from build123d import *

# Parameters (mm, degrees)
SKETCH1_R           = 101.6
SKETCH1_R_2         = 98.425
BOSS_EXTRUDE1_DEPTH = 152.4
CUT_EXTRUDE1_DEPTH  = 152.4
FILLET1_R           = 12.7


with BuildPart() as part:
    # Sketch1 → Boss-Extrude1 (new body)
    with BuildSketch(Plane(origin=(0, 0, 0), x_dir=(1, 0, 0), z_dir=(0, 1, 0))):
        Circle(SKETCH1_R)
        Circle(SKETCH1_R_2, mode=Mode.SUBTRACT)
    extrude(amount=BOSS_EXTRUDE1_DEPTH)

    # Sketch2 → Cut-Extrude1 (cut)
    with BuildSketch(Plane(origin=(0, 0, 0), x_dir=(1, 0, 0), z_dir=(0, 1, 0))):
        Polygon((570.652570484, -39.903914981), (101.352507506, -7.087257732), (0, 0), (-101.352507506, -7.087257732), (-570.652570484, -39.903914981), (-570.652570484, -980.796006784), (570.652570484, -980.796006784), align=None)
    extrude(amount=CUT_EXTRUDE1_DEPTH, mode=Mode.SUBTRACT)

    # Fillet1
    fillet1_edges = [part.edges().sort_by_distance(p)[0] for p in [
        (-99.768874577, 0, 6.97651933),
        (99.768874577, 152.4, 6.97651933),
        (-99.768874577, 152.4, 6.97651933),
        (99.768874577, 0, 6.97651933),
    ]]
    fillet(fillet1_edges, radius=FILLET1_R)


solid = part.part
CAD build for the part. Positions are in the model's coordinates, mm. A direction names the side the tool comes from. Round coordinates to 2 decimals unless told otherwise and drop trailing zeros. Loops run counter-clockwise (first coordinate to the right, second up) from the corner with the lowest first, then second, coordinate; pieces in that order, holes last.
(1) Drop flat-ended pins along their axis: pin 1 (1.5 mm diameter, centred on x = 20, y = 21, fed in from -Z); pin 2 (12 mm diameter, centred on y = 111.5, z = -71.5, fed in from +X); pin 3 (2 mm diameter, centred on y = 131.5, z = -45, fed in from -X); pin 4 (6 mm diameter, centred on x = 41.5, z = -83, fed in from -Y). Give the stop position or say it passes through.
(2) Wall check: line 1 along X through (y, z) = (78, -63); line 2 along X through (y, z) = (106, -71); line 3 along Z through (x, y) = (-43, 81.5). Give the ranges that are in metal, low to high.
(3) Which spindle directions (+Z, -Z, +X, -X, +Y, -Y) get a long thin tool onto all of the face, cutting with end or side? Do faces 1 (the flat face through (-8, 0, -100)), 2 (the cylindrical face through (-99.64, 3.82, 3.34)), 3 (the cylindrical face through (-99.64, 148.58, 3.34)). Say none if no direction does.
(4) Cut at A-A (z = -50). Give the cut face in (x, y), plus the area to 3 significant figures.
(5) Cut at D-D (z = -18.5). Give the cut face in (x, y), plus the area to 3 significant figures.
Findings below:
1. pin 1: stops at z = -99.76
1. pin 2: stops at x = 77.67
1. pin 3: stops at x = -91.58
1. pin 4: passes through
2. line 1: x = -79.71 to -75.62, 75.62 to 79.71
2. line 2: x = -72.67 to -68.17, 68.17 to 72.67
2. line 3: z = -92.05 to -88.54
3. face 1: +Z, -Z, +X, -X, -Y
3. face 2: +Z, -Y
3. face 3: +Z, +Y
4. outline: (-88.45, 0) - (-84.78, 0) - (-84.78, 152.4) - (-88.45, 152.4) - close; (84.78, 0) - (88.45, 0) - (88.45, 152.4) - (84.78, 152.4) - close
4. area: 1,120 mm2
5. outline: (-99.9, 0) - (-96.67, 0) - (-96.67, 152.4) - (-99.9, 152.4) - close; (96.67, 0) - (99.9, 0) - (99.9, 152.4) - (96.67, 152.4) - close
5. area: 985 mm2
